```python
from build123d import *

# Parameters (mm, degrees)
F0_R     = 30.48
F0_R_2   = 6.9999987
F1_DEPTH = 10.16
F2_R     = 5.07999
F3_SIZE  = 1.27


# Not quite as in the source:
# - a fillet or chamfer is up to 0.001 mm smaller than in the source, because OpenCascade refuses the exact size


with BuildPart() as f1:
    # F0 (on Top) → F1 (new body)
    with BuildSketch(Plane.XY):
        Circle(F0_R)
        Circle(F0_R_2, mode=Mode.SUBTRACT)
    extrude(amount=F1_DEPTH)

    # F2 (radius 5.08 in the source; OpenCascade refuses exactly that, so slightly less here)
    f2_edges = [f1.edges().sort_by_distance(p)[0] for p in [
        (-30.48, 0, 10.16),
        (-30.48, 0, 0),
    ]]
    fillet(f2_edges, radius=F2_R)

    # F3
    f3_edges = [f1.edges().sort_by_distance(p)[0] for p in [
        (-6.999999, 0, 10.16),
        (-6.999999, 0, 0),
    ]]
    chamfer(f3_edges, length=F3_SIZE)


solid = f1.part
```
Here's how the part is built. I have some questions about the finished solid (model axes, mm). Round coordinates to 2 decimals unless told otherwise and drop trailing zeros. Order: outer loops, then holes, each group sorted by start corner. A loop starts at its lowest first (then second) coordinate and runs counter-clockwise, first axis right, second up. Notation, with made-up numbers: M -34.5,48.5 L 21.5,48.5 A16 ccw 21.5,75.5 Z; hole C 89.25,-18 d9. An arc over 180 degrees is marked long. One line per question, with ' | ' between items.
1) If we mould it in two halves opening along X, with no side actions, what happens to faces 1 (the face through (-6, 6, 0)), 2 (the face through (3.23, -6.21, 5.03))? For each: +X half, -X half, draft (parallel to the pull), parting line (faces both ways), or undercut.
Working result:
face 1: draft | face 2: undercut
2) I want a section at C-C, the plane z = 7.75. Write out the boundary of the cut face in (x, y), then the cut area to 3 significant figures.
Working result:
outline: C 0,0 d59.44; hole C 0,0 d14 | area: 2,620 mm²
3) I need wall thicknesses on line 1 along Y through (x, z) = (4, 5.25); line 2 along Y through (x, z) = (0, 6.25); line 3 along X through (y, z) = (-0.5, 7). Which ranges of each line are inside material? Lowest first, please.
Working result:
line 1: -30.21 to -5.74, 5.74 to 30.21 | line 2: -30.34 to -7, 7 to 30.34 | line 3: -30.1 to -6.98, 6.98 to 30.1
4) I want a section at D-D, the plane z = 3.25. Write out the boundary of the cut face in (x, y).
Working result:
outline: C 0,0 d60.28; hole C 0,0 d14
5) For pin 1 Ø2 at (y, z) = (-18, 3) entering from -X; pin 2 Ø1 at (y, z) = (-5.5, 8.5) entering from -X; pin 3 Ø1 at (x, z) = (-11.5, 2) entering from +Y, each with a flat end and sliding along its axis, tell me the tip position at first contact or that it passes through.
Working result:
pin 1: x = -24.9 | pin 2: x = -29.05 | pin 3: y = 27.53
